from build123d import *

# Parameters (mm, degrees)
BASPROSKE_W     = 5.5
BASPROSKE_H     = 7.5
TOOTHCUT_DEPTH  = 12.947803145
TEETHCUTS_COUNT = 10
TEETHCUTS_ANGLE = 324
BORSKE_R        = 3.1
BORE_DEPTH      = 50.0000508
EXTRUDE_START   = -5.5
SKETCH_1_R      = 1.25
EXTRUDE_1_DEPTH = 5.5


with BuildPart() as part:
    # BasProSke → Base-Revolve (revolve)
    with BuildSketch(Plane(origin=(0, 0, 0), x_dir=(1, 0, 0), z_dir=(0, 1, 0)), mode=Mode.PRIVATE) as base_revolve_sk:
        with Locations((2.75, 3.75)):
            Rectangle(BASPROSKE_W, BASPROSKE_H)
    revolve(base_revolve_sk.sketch.rotate(Axis((-10, 0, 0), (1, 0, 0)), 180), axis=Axis((-10, 0, 0), (1, 0, 0)))

    # TooCutSke → ToothCut (cut, through all)
    with BuildSketch(Plane(origin=(0, 0, 0), x_dir=(0, 0, -1), z_dir=(1, 0, 0))):
        with BuildLine():
            ThreePointArc((0.737676151, 4.628079099), (0, 4.6865), (-0.737676151, 4.628079099))
            ThreePointArc((-0.737676151, 4.628079099), (-1.051542781, 6.151798382), (-2.205760267, 7.194877817))
            ThreePointArc((-2.205760267, 7.194877817), (0, 7.5254), (2.205760267, 7.194877817))
            ThreePointArc((2.205760267, 7.194877817), (1.051542781, 6.151798382), (0.737676151, 4.628079099))
        make_face()
    toothcut = extrude(amount=TOOTHCUT_DEPTH, mode=Mode.SUBTRACT)

    # TeethCuts: ToothCut ×10 about axis
    teethcuts_axis = Axis((-10, 0, 0), (1, 0, 0))
    for i in range(1, TEETHCUTS_COUNT):
        add(toothcut.rotate(teethcuts_axis, i * TEETHCUTS_ANGLE / (TEETHCUTS_COUNT - 1)), mode=Mode.SUBTRACT)

    # BorSke → Bore (cut, symmetric)
    with BuildSketch(Plane(origin=(0, 0, 0), x_dir=(0, 0, -1), z_dir=(1, 0, 0))):
        with Locations(Location((0, 0, 0), (0, 0, 180))):
            Circle(BORSKE_R)
    extrude(amount=BORE_DEPTH, both=True, mode=Mode.SUBTRACT)

    # ｽｹｯﾁ1 → ﾎﾞｽ - 押し出し1 (add)
    with BuildSketch(Plane(origin=(5.5, 0, 0), x_dir=(0, 0, -1), z_dir=(1, 0, 0)).offset(EXTRUDE_START)):
        with BuildLine():
            Line((2.625065975, -5), (24, -5))
            Line((24, -5), (24, 5))
            Line((24, 5), (2.625065975, 5))
            ThreePointArc((2.625065975, 5), (2.414263067, 4.564514712), (2.123524099, 4.177789805))
            ThreePointArc((2.123524099, 4.177789805), (2.754655585, 3.791458144), (3.317109183, 3.31059948))
            ThreePointArc((3.317109183, 3.31059948), (4.449153618, 4.350870864), (5.975877892, 4.53198449))
            ThreePointArc((5.975877892, 4.53198449), (6.067627458, 4.408389392), (6.156821206, 4.282937385))
            ThreePointArc((6.156821206, 4.282937385), (5.512788165, 2.886903504), (4.173610318, 2.131726803))
            ThreePointArc((4.173610318, 2.131726803), (4.457126364, 1.448208144), (4.629519252, 0.728583383))
            ThreePointArc((4.629519252, 0.728583383), (6.156818616, 0.904781587), (7.498420418, 0.153919576))
            ThreePointArc((7.498420418, 0.153919576), (7.5, 0), (7.498420418, -0.153919576))
            ThreePointArc((7.498420418, -0.153919576), (6.156818616, -0.904781587), (4.629519252, -0.728583383))
            ThreePointArc((4.629519252, -0.728583383), (4.457126364, -1.448208144), (4.173610318, -2.131726803))
            ThreePointArc((4.173610318, -2.131726803), (5.512788165, -2.886903504), (6.156821206, -4.282937385))
            ThreePointArc((6.156821206, -4.282937385), (6.067627458, -4.408389392), (5.975877892, -4.53198449))
            ThreePointArc((5.975877892, -4.53198449), (4.449153618, -4.350870864), (3.317109183, -3.31059948))
            ThreePointArc((3.317109183, -3.31059948), (2.754655585, -3.791458144), (2.123524099, -4.177789805))
            ThreePointArc((2.123524099, -4.177789805), (2.414263067, -4.564514712), (2.625065975, -5))
        make_face()
        with Locations((13, 0)):
            Circle(SKETCH_1_R, mode=Mode.SUBTRACT)
        with Locations((21, 0)):
            Circle(SKETCH_1_R, mode=Mode.SUBTRACT)
    extrude(amount=EXTRUDE_1_DEPTH)


solid = part.part
The model under review builds one solid part; all positions refer to its coordinate system, in mm. Round coordinates to 2 decimals unless told otherwise and drop trailing zeros. Order: outer loops, then holes, each group sorted by start corner. A loop starts at its lowest first (then second) coordinate and runs counter-clockwise, first axis right, second up. Notation, with made-up numbers: (31, -38) -> (55, -38) arc R15 cw to (55, -14) -> close; hole circle Ø11 at (-11, 45). An arc over 180 degrees is marked (long way). Return JSON: item names as keys, results as strings.
1. The part is to be moulded in two halves that separate along Y. For faces 1 (the face through (2.71, 0.91, 6.14)), 2 (the face through (5.5, 0.1, -11.5)), say which applies: +Y half, -Y half, draft (parallel to the pull), parting line (faces both ways), or undercut.
Answer block:
{"face 1": "undercut", "face 2": "draft"}
2. Insertion check: P1, Ø2, axis at y = 0, z = -21, coming from the -X side; P2, Ø1.6, axis at x = 2, z = -17.5, coming from the +Y side; P3, Ø2, axis at x = 2, y = 3.5, coming from the +Z side. Each pin has a flat end and moves straight along its axis. Give the tip position at first contact, or say it passes through.
Answer block:
{"P1": "passes through", "P2": "stops at y = 5", "P3": "stops at z = 6.16"}
3. Take a section at D-D (z = 5.5). Write out the cut boundary in (x, y), then the cut area to 3 significant figures.
Answer block:
{"outline": "(0, -4.58) -> (5.5, -4.58) -> (5.5, -2.87) -> (0, -2.87) -> close; (0, -0.95) -> (5.5, -0.95) -> (5.5, 0.95) -> (0, 0.95) -> close; (0, 2.87) -> (5.5, 2.87) -> (5.5, 4.58) -> (0, 4.58) -> close", "area": "29.2 mm²"}
4. Take a section at C-C (z = -21). Write out the cut boundary in (x, y), then the cut area to 4 significant figures.
Answer block:
{"outline": "(0, -5) -> (5.5, -5) -> (5.5, -1.25) -> (0, -1.25) -> close; (0, 1.25) -> (5.5, 1.25) -> (5.5, 5) -> (0, 5) -> close", "area": "41.25 mm²"}
5. Take a section at B-B (x = 1.45). State how many separate pieces and enclosed holes the cut face has, then the cut area to 3 significant figures.
Answer block:
{"separate pieces": "1", "enclosed holes": "3", "area": "262 mm²"}
6. Take a section at A-A (z = 0). Write out the cut boundary in (x, y).
Answer block:
{"outline": "(0, -4.69) -> (5.5, -4.69) -> (5.5, -3.1) -> (0, -3.1) -> close; (0, 3.1) -> (5.5, 3.1) -> (5.5, 4.69) -> (0, 4.69) -> close"}
7. For L1, parallel to Y at x = 2.95, z = 0; L2, parallel to Y at x = 3.05, z = -21; L3, parallel to Y at x = 3, z = -5.5, list the stretches that pass through material, from the lowest coordinate up. Write a range as [from, to].
Answer block:
{"L1": "y = [-4.69, -3.1], [3.1, 4.69]", "L2": "y = [-5, -1.25], [1.25, 5]", "L3": "y = [-5, 5]"}
